Verification items for the finished model (mm, model axes). Round coordinates to 2 decimals unless told otherwise and drop trailing zeros. Order: outer loops, then holes, each group sorted by start corner. A loop starts at its lowest first (then second) coordinate and runs counter-clockwise, first axis right, second up. Notation, with made-up numbers: M 14,-21.5 L 54,-21.5 A36 cw 54,12.5 Z; hole C 33,72 d8. An arc over 180 degrees is marked long. Use CSV: the item, a comma, the result in double quotes. Start each with the question number.
Q1. Sectioned sample at C-C (z = 12). Enter the section's corners in (x, y), and give its area (3 significant figures).
Q2. Sectioned sample at A-A (z = 0). Enter the section's corners in (x, y), and give its area (3 significant figures).
Q3. Gauge pin test, flat ends, axial feed: pin 1 Ø11 at (x, z) = (-8.63, 26.57) entering from +Y; pin 2 Ø6 at (x, z) = (-8.63, -26.57) entering from -Y; pin 3 Ø3 at (x, y) = (-2.5, 5.5) entering from -Z; pin 4 Ø3 at (y, z) = (0.5, 10) entering from -X. Record the tip position at first contact, or that the pin passes through.
Q4. Mould release check, pull along Z, two halves, no side actions. Record for faces 1 (the face through (13, 6.35, -15)), 2 (the face through (-11.081, 3.131, 34.337)), 3 (the face through (-11.2, 3.1, -34.3)), 4 (the face through (-10.45, 3.131, 23.724)): +Z half, -Z half, draft (parallel to the pull), parting line (faces both ways), or undercut.
Q5. Sectioned sample at D-D (y = 3.75). Enter the section's corners in (x, z) (1 decimal), and give its area (3 significant figures).
Q6. Scan lines: line 1 (X direction, y = 5, z = 17.5); line 2 (X direction, y = 0.75, z = 15); line 3 (Z direction, x = -29.5, y = 2.25). Record each from-to range of solid material in increasing order.
Q7. Sectioned sample at B-B (x = 5). Enter the section's corners in (y, z), and give its area (3 significant figures).
Autodesk Inventor part; units mm, degrees
ref_plane "YZ Plane" through (0, 0, 0) normal (1, 0, 0) x (0, 1, 0)
ref_plane "XZ Plane" through (0, 0, 0) normal (0, 1, 0) x (-1, 0, 0)
ref_plane "XY Plane" through (0, 0, 0) normal (0, 0, 1) x (1, 0, 0)
sketch "Sketch1" plane through (0, 0, 0) normal (0, 1, 0) x (-1, 0, 0)
  circle A0 centre (0, 0) radius 19.304
  line L0 (0, 0) -> (27.94, 0) construction
  circle A1 centre (27.94, 0) radius 3.3782
  circle A2 centre (8.6339, 26.5725) radius 3.3782
  circle A3 centre (-22.6039, 16.4227) radius 3.3782
  circle A4 centre (-22.6039, -16.4227) radius 3.3782
  circle A5 centre (8.6339, -26.5725) radius 3.3782
  line L1 (34.526, 4.785) -> (15.2199, 31.3575)
  arc A6 (15.2199, 31.3575) -> (6.1183, 34.3148) centre (8.6339, 26.5725) ccw
  line L2 (6.1183, 34.3148) -> (-25.1195, 24.165)
  arc A7 (-25.1195, 24.165) -> (-30.7446, 16.4227) centre (-22.6039, 16.4227) ccw
  line L3 (-30.7446, 16.4227) -> (-30.7446, -16.4227)
  arc A8 (-30.7446, -16.4227) -> (-25.1195, -24.165) centre (-22.6039, -16.4227) ccw
  line L4 (-25.1195, -24.165) -> (6.1183, -34.3148)
  arc A9 (6.1183, -34.3148) -> (15.2199, -31.3575) centre (8.6339, -26.5725) ccw
  line L5 (15.2199, -31.3575) -> (34.526, -4.785)
  arc A10 (34.526, -4.785) -> (34.526, 4.785) centre (27.94, 0) ccw
  dimension "d0" = 38.608
  dimension "d1" = 27.94
  dimension "d2" = 6.7564
  dimension "d5" = 360
  dimension "d7" = 4.7625
extrude "Extrusion1" add sketch "Sketch1" along normal blind 6.35
properties part number "gearSpacer" material "Aluminum 6061"
Verdict:
1,outline,"M -29.28,0 L -15.12,0 L -15.12,6.35 L -29.28,6.35 Z; M 15.12,0 L 30.74,0 L 30.74,6.35 L 15.12,6.35 Z"
1,area,"189 mm²"
2,outline,"M -36.08,0 L -31.32,0 L -31.32,6.35 L -36.08,6.35 Z; M -24.56,0 L -19.3,0 L -19.3,6.35 L -24.56,6.35 Z; M 19.3,0 L 30.74,0 L 30.74,6.35 L 19.3,6.35 Z"
2,area,"136 mm²"
3,pin 1,"stops at y = 6.35"
3,pin 2,"passes through"
3,pin 3,"stops at z = -33.63"
3,pin 4,"stops at x = -31.83"
4,face 1,"draft"
4,face 2,"+Z half"
4,face 3,"-Z half"
4,face 4,"undercut"
5,outline,"M -34.5,-4.8 L -15.2,-31.4 A8.1 ccw -6.1,-34.3 L 25.1,-24.2 A8.1 ccw 30.7,-16.4 L 30.7,16.4 A8.1 ccw 25.1,24.2 L -6.1,34.3 A8.1 ccw -15.2,31.4 L -34.5,4.8 A8.1 ccw Z; hole C -27.9,0 d6.8; hole C 0,0 d38.6; hole C -8.6,-26.6 d6.8; hole C -8.6,26.6 d6.8; hole C 22.6,-16.4 d6.8; hole C 22.6,16.4 d6.8"
5,area,"2,050 mm²"
6,line 1,"x = -25.29 to -8.15, 8.15 to 19.4, 25.81 to 30.67"
6,line 2,"x = -27.1 to -12.15, 12.15 to 19.54, 25.67 to 30.74"
6,line 3,"z = -11.7 to -3, 3 to 11.7"
7,outline,"M 0,-30.7 L 6.35,-30.7 L 6.35,-18.65 L 0,-18.65 Z; M 0,18.65 L 6.35,18.65 L 6.35,30.7 L 0,30.7 Z"
7,area,"153 mm²"
